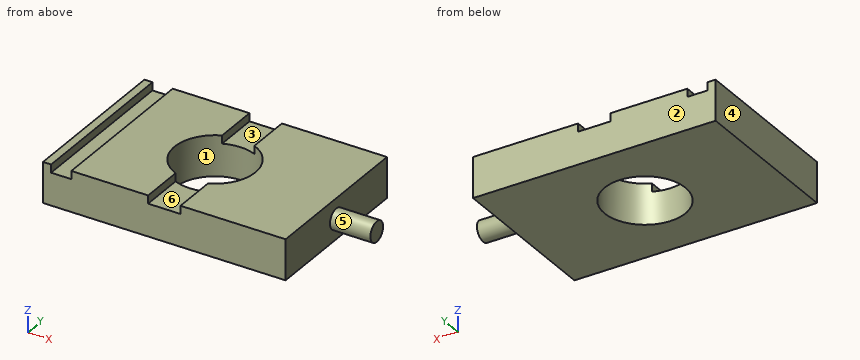
```python
from build123d import *

# Parameters (mm, degrees)
F0_W     = 76.2
F0_H     = 50.8
F0_R     = 12.7
F1_DEPTH = 12.7
F2_W     = 6.35
F2_H     = 50.8
F3_DEPTH = 2.54
F4_R     = 3.175
F5_DEPTH = 12.7


with BuildPart() as f1:
    # F0 (on Top) → F1 (new body)
    with BuildSketch(Plane.XY):
        Rectangle(F0_W, F0_H)
        Circle(F0_R, mode=Mode.SUBTRACT)
    extrude(amount=F1_DEPTH)

    # F2 (on face) → F3 (cut)
    with BuildSketch(Plane.XY.offset(12.7)):
        with Locations((-32.385, 0)):
            Rectangle(F2_W, F2_H)
        with BuildLine():
            Line((5.08, 25.4), (-5.08, 25.4))
            Line((-5.08, 25.4), (-5.08, 11.639742))
            ThreePointArc((-5.08, 11.639742), (0, 12.7), (5.08, 11.639742))
            Line((5.08, 11.639742), (5.08, 25.4))
        make_face()
        with BuildLine():
            Line((-5.08, -11.639742), (-5.08, -25.4))
            Line((-5.08, -25.4), (5.08, -25.4))
            Line((5.08, -25.4), (5.08, -11.639742))
            ThreePointArc((5.08, -11.639742), (0, -12.7), (-5.08, -11.639742))
        make_face()
    extrude(amount=-F3_DEPTH, mode=Mode.SUBTRACT)

    # F4 (on face) → F5 (join)
    with BuildSketch(Plane.YZ.offset(38.1)):
        with Locations((0, 6.35)):
            Circle(F4_R)
    extrude(amount=F5_DEPTH)


solid = f1.part
```
Could you check a few things on this model? Use its own coordinates, in mm. Face numbers are marked on the shaded views. A direction names the side the tool comes from. Give positions to 0.01 mm unless a question says otherwise; leave off trailing zeros. Order: outer loops, then holes, each group sorted by start corner. A loop starts at its lowest first (then second) coordinate and runs counter-clockwise, first axis right, second up.
Q1. Suppose I cut it at C-C, the plane y = 0. Write out the boundary of the cut face in (x, z) (3 decimals), and give its area (3 significant figures).
Q2. Suppose I cut it at D-D, the plane z = 2. Write out the boundary of the cut face in (x, y).
Q3. Suppose I cut it at A-A, the plane z = 11.75. Write out the boundary of the cut face in (x, y).
Q4. I'm going to push flat-ended pins straight in: P1, Ø3, axis at y = -16.5, z = 11, coming from the +X side; P2, Ø8, axis at x = 1, y = 18, coming from the +Z side. Where does each tip first touch, or does it pass through?
Q5. Suppose I cut it at B-B, the plane x = 0. Write out the boundary of the cut face in (y, z), and give its area (3 significant figures).
Q6. If I drill on line 1 along X through (y, z) = (17, 10.25); line 2 along X through (y, z) = (0, 4.25); line 3 along X through (y, z) = (0, 2.5), over which ranges is the centre line in solid material (lowest first)?
Q7. We'd pull the mould along Y, two halves only. Please class the marked faces 1, 2 and 3: +Y half, -Y half, draft (parallel to the pull), parting line (faces both ways), or undercut.
Q8. For the marked faces 4, 5 and 6, which set-ups out of +Z, -Z, +X, -X, +Y, -Y let a thin tool reach every point of the face, with its end or its side?
Solution:
1. outline: (-38.1, 0) - (-12.7, 0) - (-12.7, 12.7) - (-29.21, 12.7) - (-29.21, 10.16) - (-35.56, 10.16) - (-35.56, 12.7) - (-38.1, 12.7) - close; (12.7, 0) - (38.1, 0) - (38.1, 3.175) - (50.8, 3.175) - (50.8, 9.525) - (38.1, 9.525) - (38.1, 12.7) - (12.7, 12.7) - close
1. area: 710 mm2
2. outline: (-38.1, -25.4) - (38.1, -25.4) - (38.1, 25.4) - (-38.1, 25.4) - close; hole circle Ø25.4 at (0, 0)
3. outline: (-38.1, -25.4) - (-35.56, -25.4) - (-35.56, 25.4) - (-38.1, 25.4) - close; (-29.21, -25.4) - (-5.08, -25.4) - (-5.08, -11.64) arc R12.7 cw to (-5.08, 11.64) - (-5.08, 25.4) - (-29.21, 25.4) - close; (5.08, -25.4) - (38.1, -25.4) - (38.1, 25.4) - (5.08, 25.4) - (5.08, 11.64) arc R12.7 cw to (5.08, -11.64) - close
4. P1: stops at x = 38.1
4. P2: stops at z = 10.16
5. outline: (-25.4, 0) - (-12.7, 0) - (-12.7, 10.16) - (-25.4, 10.16) - close; (12.7, 0) - (25.4, 0) - (25.4, 10.16) - (12.7, 10.16) - close
5. area: 258 mm2
6. line 1: x = -38.1 to -35.56, -29.21 to -5.08, 5.08 to 38.1
6. line 2: x = -38.1 to -12.7, 12.7 to 50.8
6. line 3: x = -38.1 to -12.7, 12.7 to 38.1
7. face 1: undercut
7. face 2: +Y half
7. face 3: draft
8. face 4: +Z, -Z, -X, +Y, -Y
8. face 5: +X
8. face 6: +Z, +Y, -Y
